```python
from build123d import *

# Parameters (mm, degrees)
F0_W     = 159
F0_H     = 100
F1_DEPTH = 4
F2_W     = 31.5
F2_H     = 4
F3_DEPTH = 4
F4_W     = 4
F4_H     = 25
F5_DEPTH = 4
F6_W     = 4
F6_H     = 50
F7_DEPTH = 4


with BuildPart() as f1:
    # F0 (on Top) → F1 (new body)
    with BuildSketch(Plane.XY):
        with Locations((79.5, 50)):
            Rectangle(F0_W, F0_H)
    extrude(amount=F1_DEPTH)

    # F2 (on face) → F3 (cut, through all)
    with BuildSketch(Plane.XY.offset(4)):
        with Locations((47.75, 2)):
            Rectangle(F2_W, F2_H)
        with Locations((111.25, 2)):
            Rectangle(F2_W, F2_H)
    extrude(amount=-F3_DEPTH, mode=Mode.SUBTRACT)

    # F4 (on face) → F5 (cut, through all)
    with BuildSketch(Plane.XY.offset(4)):
        with Locations((157, 12.5)):
            Rectangle(F4_W, F4_H)
        with Locations((157, 87.5)):
            Rectangle(F4_W, F4_H)
        with Locations((2, 87.5)):
            Rectangle(F4_W, F4_H)
        with Locations((2, 12.5)):
            Rectangle(F4_W, F4_H)
    extrude(amount=-F5_DEPTH, mode=Mode.SUBTRACT)

    # F6 (on face) → F7 (cut, through all)
    with BuildSketch(Plane.XY.offset(4)):
        with Locations((79.5, 50)):
            Rectangle(F6_W, F6_H)
    extrude(amount=-F7_DEPTH, mode=Mode.SUBTRACT)


solid = f1.part
```
Can you work these out from the model? Positions are in its coordinate system, mm. A direction names the side the tool comes from. Give positions to 0.01 mm unless a question says otherwise; leave off trailing zeros. Loops run counter-clockwise (first coordinate to the right, second up) from the corner with the lowest first, then second, coordinate; pieces in that order, holes last. Notation, with made-up numbers: M 45,-38 L 93,-38 A6 ccw 93,-29 Z; hole C 56,48.5 d1. An arc over 180 degrees is marked long. One line per item, written item: value.
(1) I need wall thicknesses on line 1 (X direction, y = 72, z = 3.85); line 2 (X direction, y = 16.5, z = 0.6); line 3 (Y direction, x = 50, z = 0.3). Which ranges of each line are inside material? Lowest first, please.
Returned:
line 1: 0 to 77.5, 81.5 to 159
line 2: 4 to 155
line 3: 4 to 100
(2) Suppose I cut it at A-A on y = 46. List the corners of the cut face in (x, z) for me.
Returned:
outline: M 0,0 L 77.5,0 L 77.5,4 L 0,4 Z; M 81.5,0 L 159,0 L 159,4 L 81.5,4 Z
(3) Suppose I cut it at B-B on z = 1.6. List the corners of the cut face in (x, y) for me, plus the area to 3 significant figures.
Returned:
outline: M 0,25 L 4,25 L 4,0 L 32,0 L 32,4 L 63.5,4 L 63.5,0 L 95.5,0 L 95.5,4 L 127,4 L 127,0 L 155,0 L 155,25 L 159,25 L 159,75 L 155,75 L 155,100 L 4,100 L 4,75 L 0,75 Z; hole M 77.5,25 L 81.5,25 L 81.5,75 L 77.5,75 Z
area: 15,000 mm^2
(4) Suppose I cut it at D-D on y = 15. List the corners of the cut face in (x, z) for me.
Returned:
outline: M 4,0 L 155,0 L 155,4 L 4,4 Z
(5) Will these pins go through, and if not, where does the flat tip stop? pin 1 (1.2 mm diameter, centred on x = 80, z = 2.5, fed in from -Y); pin 2 (1.2 mm diameter, centred on x = 55, z = 1.5, fed in from -Y); pin 3 (1.2 mm diameter, centred on y = 86.5, z = 1.5, fed in from +X); pin 4 (2 mm diameter, centred on y = 89.5, z = 1.5, fed in from -X).
Returned:
pin 1: y = 0
pin 2: y = 4
pin 3: x = 155
pin 4: x = 4
(6) Which directions (+Z, -Z, +X, -X, +Y, -Y) give clear straight access to the entire face, cutting with the end or side of a thin tool? Please do faces 1 (the face through (155, 12, 2)), 2 (the face through (81.5, 50, 2)), 3 (the face through (111, 4, 2)).
Returned:
face 1: +Z, -Z, +X, -Y
face 2: +Z, -Z
face 3: +Z, -Z, -Y
(7) Suppose I cut it at C-C on x = 52.5. List the corners of the cut face in (y, z) for me.
Returned:
outline: M 4,0 L 100,0 L 100,4 L 4,4 Z
(8) We'd pull the mould along Y, two halves only. Please class faces 4 (the face through (61, 51, 0)), 5 (the face through (79, 25, 2)), 6 (the face through (18, 0, 2)), 7 (the face through (78, 100, 2)): released by +Y, released by -Y, zero draft, split by the parting line, or undercut.
Returned:
face 4: zero draft
face 5: undercut
face 6: released by -Y
face 7: released by +Y
